The drawing under review shows one solid part. Ordinate dimensions are in mm from its lowest x, y, z. Coordinates: 2 decimals unless noted, no trailing zeros. Loops run counter-clockwise (first coordinate to the right, second up) from the corner with the lowest first, then second, coordinate; pieces in that order, holes last. Notation, with made-up numbers: M 61,63 L 70,63 A31 ccw 70,96 Z; hole C -20,11.25 d10. An arc over 180 degrees is marked long. Return JSON: item names as keys, results as strings.
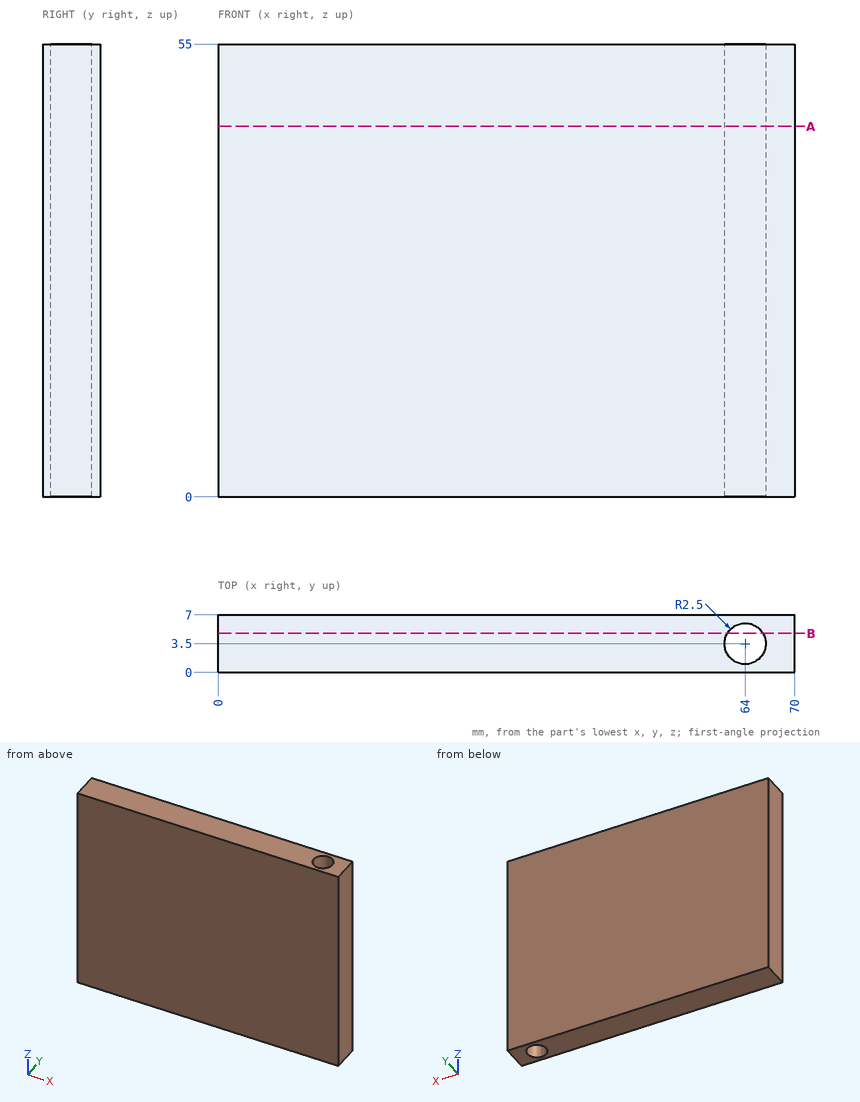
1. Add section A-A on z = 45. Give the boundary of the cut face in (x, y), plus the area to 3 significant figures.
Check values:
{"outline": "M 0,0 L 70,0 L 70,7 L 0,7 Z; hole C 64,3.5 d5", "area": "470 mm²"}
2. Insertion check: pin 1 Ø1 at (x, z) = (58, 41) entering from -Y. The pin has a flat end and moves straight along its axis. Give the tip position at first contact, or say it passes through.
Check values:
{"pin 1": "y = 0"}
3. To check wall thickness, follow line 1 (X direction, y = 3.5, z = 40.5); line 2 (X direction, y = 5, z = 25); line 3 (Y direction, x = 66, z = 17). State the ranges of each line that lie inside material, in increasing order.
Check values:
{"line 1": "0 to 61.5, 66.5 to 70", "line 2": "0 to 62, 66 to 70", "line 3": "0 to 2, 5 to 7"}
4. Add section B-B on y = 4.75. Give the boundary of the cut face in (x, z), plus the area to 3 significant figures.
Check values:
{"outline": "M 0,0 L 61.83,0 L 61.83,55 L 0,55 Z; M 66.17,0 L 70,0 L 70,55 L 66.17,55 Z", "area": "3,610 mm²"}
